Read the model definition and answer for the solid it produces. Units are mm, in the model's axes. Face numbers are marked on the shaded views. A direction names the side the tool comes from. Give positions to 0.01 mm unless a question says otherwise; leave off trailing zeros. Loops run counter-clockwise (first coordinate to the right, second up) from the corner with the lowest first, then second, coordinate; pieces in that order, holes last. Notation, with made-up numbers: (86, 71) -> (121, 71) arc R4 cw to (121, 75) -> close; hole circle Ø4 at (31, 47). An arc over 180 degrees is marked (long way). One line per item, written item: value. Start each with the question number.
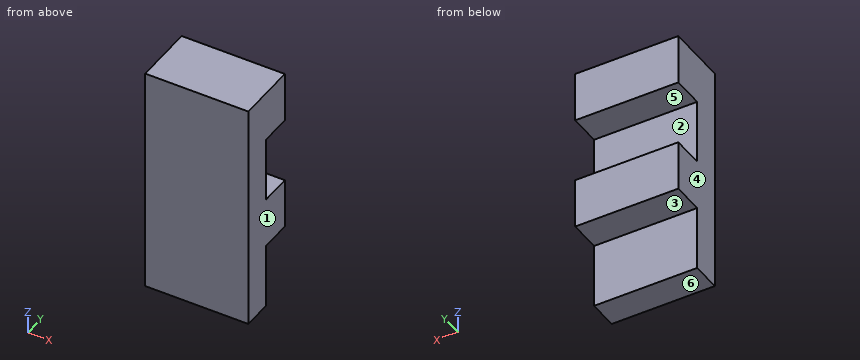
from build123d import *

# Parameters (mm, degrees)
BOSS_EXTRUDE1_DEPTH = 9.8
LPATTERN1_COUNT     = 2
LPATTERN1_PITCH     = 11


with BuildPart() as part:
    # Sketch1 → Boss-Extrude1 (new body)
    with BuildSketch(Plane(origin=(0, 0, 0), x_dir=(0, 0, -1), z_dir=(1, 0, 0))):
        Polygon((0, 0), (4.8, 0), (11, 0), (11, 2.8), (4.8, 2.8), (4.8, 5.8), (0, 5.8), align=None)
    boss_extrude1 = extrude(amount=BOSS_EXTRUDE1_DEPTH)

    # LPattern1: Boss-Extrude1 ×2
    with Locations(*[(0, 0, -i * LPATTERN1_PITCH) for i in range(1, LPATTERN1_COUNT)]):
        add(boss_extrude1)


solid = part.part
Item 1: Section A-A, the plane y = 3.8 is taken. Determine the outline of the cut face in (x, z).
Item 2: Section B-B, the plane x = 4 is taken. Determine the outline of the cut face in (y, z).
Item 3: Consider L1, parallel to Z at x = 2.5, y = 4.65; L2, parallel to Y at x = 7.5, z = -16.75. Determine where each line is inside the solid, lowest interval first. Write a range as [from, to].
Item 4: For the marked faces 1, 2 and 3, determine the directions among +Z, -Z, +X, -X, +Y, -Y from which every point of the face is accessible in a straight line to the end or side of a thin tool.
Item 5: Flat-ended cylindrical pins translate along their axes: pin 1 (5 mm diameter, centred on x = 6.5, z = -19.5, fed in from +Y); pin 2 (1 mm diameter, centred on x = 1.5, y = 3, fed in from +Z); pin 3 (1.5 mm diameter, centred on x = 1, y = 4, fed in from -Z). Find the tip coordinate at first contact, or state that the pin passes through.
Item 6: Determine the mould class of the marked faces 4, 5 and 6 for opening direction Z: pulls with the +Z half, pulls with the -Z half, needs draft (parallel to the pull), parting line crosses it, or undercut.
Item 7: Section C-C, the plane z = -19.25 is taken. Determine the outline of the cut face in (x, y), plus the area to 3 significant figures.
Computed values:
1. outline: (0, -15.8) -> (9.8, -15.8) -> (9.8, -11) -> (0, -11) -> close; (0, -4.8) -> (9.8, -4.8) -> (9.8, 0) -> (0, 0) -> close
2. outline: (0, -22) -> (2.8, -22) -> (2.8, -15.8) -> (5.8, -15.8) -> (5.8, -11) -> (2.8, -11) -> (2.8, -4.8) -> (5.8, -4.8) -> (5.8, 0) -> (0, 0) -> close
3. L1: [-15.8, -11], [-4.8, 0]
3. L2: [0, 2.8]
4. face 1: +Z, -Z, +X, +Y, -Y
4. face 2: +X, -X, +Y
4. face 3: -Z, +X, -X, +Y
5. pin 1: y = 2.8
5. pin 2: z = 0
5. pin 3: z = -15.8
6. face 4: needs draft
6. face 5: undercut
6. face 6: pulls with the -Z half
7. outline: (0, 0) -> (9.8, 0) -> (9.8, 2.8) -> (0, 2.8) -> close
7. area: 27.4 mm²
